Can you work these out from the model? Positions are in its coordinate system, mm. Round coordinates to 2 decimals unless told otherwise and drop trailing zeros. Order: outer loops, then holes, each group sorted by start corner. A loop starts at its lowest first (then second) coordinate and runs counter-clockwise, first axis right, second up.
Q1. If we section it at A-A (x = 57.5): Please give me the cut outline in (y, z).
Q2. We'd pull the mould along X, two halves only. Please class faces 1 (the face through (55, 46, 0)), 2 (the face through (0, 46, 2)), 3 (the face through (16.549, 51, 2)): pulls with the +X half, pulls with the -X half, needs draft (parallel to the pull), parting line crosses it, or undercut.
Q3. If we section it at C-C (z = 3.5): Count the separate pieces of the cut face and the enclosed holes in it, plus the area to 3 significant figures.
Q4. If I drill on line 1 (Y direction, x = 81.5, z = 0.95); line 2 (X direction, y = 37, z = 1.55); line 3 (X direction, y = 29, z = 1.9), over which ranges is the centre line in solid material (lowest first)?
Q5. If we section it at B-B (x = 32.5): Please give me the cut outline in (y, z), plus the area to 3 significant figures.
Autodesk Inventor part; units mm, degrees
ref_plane "YZ Plane" through (0, 0, 0) normal (1, 0, 0) x (0, 1, 0)
ref_plane "XZ Plane" through (0, 0, 0) normal (0, 1, 0) x (-1, 0, 0)
ref_plane "XY Plane" through (0, 0, 0) normal (0, 0, 1) x (1, 0, 0)
sketch "Sketch1" plane through (0, 0, 0) normal (0, 0, 1) x (1, 0, 0)
  line L0 (0, 0) -> (111.76, 0)
  line L1 (111.76, 0) -> (111.76, 91.44)
  line L2 (111.76, 91.44) -> (0, 91.44)
  line L3 (0, 91.44) -> (0, 0)
  dimension "d0" = 111.76
  dimension "d1" = 91.44
extrude "Extrusion1" add sketch "Sketch1" along normal blind 4.826
sketch "Sketch2" plane through (0, 0, 4.826) normal (0, 0, 1) x (1, 0, 0)
  line L0 (111.76, 0) -> (111.76, 91.44)
  line L1 (34.5493, 37.338) -> (52.5493, 37.338)
  line L2 (52.5493, 40.338) -> (16.5493, 40.338)
  line L3 (16.5493, 43.338) -> (52.5493, 43.338)
  line L4 (34.5493, 46.338) -> (52.5493, 46.338)
  line L5 (16.5493, 49.338) -> (52.5493, 49.338)
  line L6 (52.5493, 52.338) -> (16.5493, 52.338)
  line L7 (34.5493, 55.338) -> (52.5493, 55.338)
  line L8 (16.5493, 58.338) -> (52.5493, 58.338)
  line L9 (16.5493, 58.338) -> (16.5493, 22.338)
  line L10 (52.5493, 22.338) -> (16.5493, 22.338)
  line L11 (34.5493, 25.338) -> (52.5493, 25.338)
  line L12 (34.5493, 28.338) -> (52.5493, 28.338)
  line L13 (34.5493, 31.338) -> (52.5493, 31.338)
  line L14 (34.5493, 34.338) -> (52.5493, 34.338)
  line L15 (66.96, 79.167) -> (86.76, 79.167)
  line L16 (66.96, 61.44) -> (66.96, 79.167)
  line L17 (86.76, 61.44) -> (66.96, 61.44)
  line L18 (86.76, 79.167) -> (86.76, 61.44)
  line L19 (60.6088, 74.0565) -> (60.6088, 65.8015)
  line L20 (60.6088, 65.8015) -> (45.0584, 65.8015)
  line L21 (45.0584, 65.8015) -> (45.0584, 74.0565)
  line L22 (45.0584, 74.0565) -> (60.6088, 74.0565)
  circle A0 centre (7.874, 25.4) radius 4.0005
  line L23 (66.96, 79.167) -> (86.76, 79.167)
  line L24 (86.76, 79.167) -> (86.76, 61.44)
  line L25 (86.76, 61.44) -> (66.96, 61.44)
  line L26 (66.96, 61.44) -> (66.96, 79.167)
  line L27 (52.5493, 58.338) -> (16.5493, 58.338)
  line L28 (16.5493, 58.338) -> (16.5493, 22.338)
  line L29 (16.5493, 22.338) -> (52.5493, 22.338)
  line L30 (52.5493, 22.338) -> (52.5493, 58.338)
  circle A1 centre (7.874, 25.4) radius 4.0005
  line L31 (34.5493, 58.338) -> (34.5493, 22.338)
  line L32 (16.5493, 55.338) -> (52.5493, 55.338)
  line L33 (52.5493, 52.338) -> (16.5493, 52.338)
  line L34 (16.5493, 49.338) -> (52.5493, 49.338)
  line L35 (52.5493, 46.338) -> (16.5493, 46.338)
  line L36 (16.5493, 43.338) -> (52.5493, 43.338)
  line L37 (52.5493, 40.338) -> (16.5493, 40.338)
  line L38 (16.5493, 37.338) -> (52.5493, 37.338)
  line L39 (52.5493, 34.338) -> (16.5493, 34.338)
  line L40 (16.5493, 31.338) -> (52.5493, 31.338)
  line L41 (52.5493, 28.338) -> (16.5493, 28.338)
  line L42 (16.5493, 25.338) -> (52.5493, 25.338)
  line L43 (60.6088, 0) -> (60.6088, 50.8)
  line L44 (111.76, 91.44) -> (111.76, 61.44)
  line L45 (111.76, 61.44) -> (86.76, 61.44)
  line L46 (86.76, 79.167) -> (86.76, 61.44)
  point P0 (0, 0)
  point P1 (0, 0)
  point P2 (0, 0)
  point P3 (0, 0)
  point P4 (0, 0)
  point P5 (16.5493, 28.338)
  dimension "d4" = 50.8
  dimension "d7" = 30
  dimension "d8" = 25
extrude "Extrusion2" cut sketch "Sketch2" against normal blind 4.826 contours L1 L30 L14 L31 | L31 L39 L9 L38 | L13 L30 L12 L31 | L31 L41 L9 L40 | L31 L4 L30 L3 | L3 L9 L35 L31 | L11 L30 L10 L31 | L31 L10 L9 L42 | L31 L6 L30 L5 | L5 L9 L6 L31 | L31 L8 L30 L7 | L32 L9 L8 L31 | L15 L18 L17 L16 | L19 L20 L21 L22 | A0
properties part number "compnent box front"
Solution:
1. outline: (0, 0) - (65.8, 0) - (65.8, 4.83) - (0, 4.83) - close; (74.06, 0) - (91.44, 0) - (91.44, 4.83) - (74.06, 4.83) - close
2. face 1: needs draft
2. face 2: pulls with the -X half
2. face 3: undercut
3. separate pieces: 1
3. enclosed holes: 9
3. area: 9,040 mm2
4. line 1: y = 0 to 61.44, 79.17 to 91.44
4. line 2: x = 0 to 16.55, 52.55 to 111.76
4. line 3: x = 0 to 6.13, 9.62 to 16.55, 52.55 to 111.76
5. outline: (0, 0) - (22.34, 0) - (22.34, 4.83) - (0, 4.83) - close; (25.34, 0) - (28.34, 0) - (28.34, 4.83) - (25.34, 4.83) - close; (31.34, 0) - (34.34, 0) - (34.34, 4.83) - (31.34, 4.83) - close; (37.34, 0) - (43.34, 0) - (43.34, 4.83) - (37.34, 4.83) - close; (46.34, 0) - (49.34, 0) - (49.34, 4.83) - (46.34, 4.83) - close; (52.34, 0) - (55.34, 0) - (55.34, 4.83) - (52.34, 4.83) - close; (58.34, 0) - (91.44, 0) - (91.44, 4.83) - (58.34, 4.83) - close
5. area: 354 mm2
